The model under review builds one solid part; all positions refer to its coordinate system, in mm. Face numbers are marked on the shaded views. A direction names the side the tool comes from. Give positions to 0.01 mm unless a question says otherwise; leave off trailing zeros. Order: outer loops, then holes, each group sorted by start corner. A loop starts at its lowest first (then second) coordinate and runs counter-clockwise, first axis right, second up. Notation, with made-up numbers: (52.25, 61.5) -> (70.25, 61.5) arc R21 cw to (70.25, 74.5) -> close; hole circle Ø7 at (39, 41.5). An arc over 180 degrees is marked (long way). Use one line per item in the form item = value.
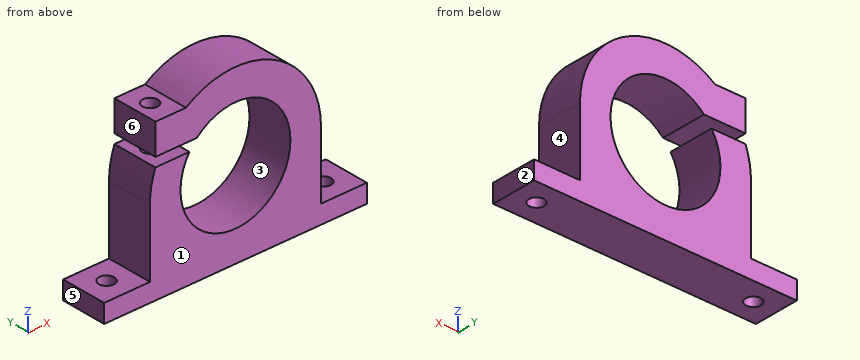
```python
from build123d import *

# Parameters (mm, degrees)
F1_DEPTH = 7.5
F2_R     = 2.5
F3_DEPTH = 6
F4_R     = 2.5
F5_DEPTH = 18


with BuildPart() as f1:
    # F0 (on Front) → F1 (new body, symmetric)
    with BuildSketch(Plane.XZ):
        with BuildLine():
            ThreePointArc((28, 0), (12.841967, 24.881396), (-16.220278, 22.823291))
            Line((-16.220278, 22.823291), (-26.220278, 22.823291))
            Line((-26.220278, 22.823291), (-26.220278, 12.823291))
            Line((-26.220278, 12.823291), (-12.631834, 12.823291))
            ThreePointArc((-12.631834, 12.823291), (13.938464, -11.389434), (-15.083201, 9.823291))
            Line((-15.083201, 9.823291), (-26.220278, 9.823291))
            ThreePointArc((-26.220278, 9.823291), (-27.551477, 4.991604), (-28, 0))
            Line((-28, 0), (-28, -22))
            Line((-28, -22), (-43, -22))
            Line((-43, -22), (-43, -28))
            Line((-43, -28), (43, -28))
            Line((43, -28), (43, -22))
            Line((43, -22), (28, -22))
            Line((28, -22), (28, 0))
        make_face()
    extrude(amount=F1_DEPTH, both=True)

    # F2 (on face) → F3 (cut, through all)
    with BuildSketch(Plane.XY.offset(-22)):
        with Locations((-35.5, 0)):
            Circle(F2_R)
        with Locations((35.5, 0)):
            Circle(F2_R)
    extrude(amount=-F3_DEPTH, mode=Mode.SUBTRACT)

    # F4 (on face) → F5 (cut)
    with BuildSketch(Plane.XY.offset(22.823291)):
        with Locations((-21.220278, 0)):
            Circle(F4_R)
    extrude(amount=-F5_DEPTH, mode=Mode.SUBTRACT)


solid = f1.part
```
1. For L1, parallel to Y at x = 35.5, z = -23.95; L2, parallel to Z at x = -16, y = -4; L3, parallel to Z at x = 4, y = 3.5, list the stretches that pass through material, from the lowest coordinate up.
Values:
L1 = -7.5 to -2.5, 2.5 to 7.5
L2 = -28 to -8.25, 8.25 to 9.82, 12.82 to 22.98
L3 = -28 to -17.55, 17.55 to 27.71
2. Add section D-D on z = 7. Give the boundary of the cut face in (x, y).
Values:
outline = (-27.11, -7.5) -> (-16.58, -7.5) -> (-16.58, 7.5) -> (-27.11, 7.5) -> close; (16.58, -7.5) -> (27.11, -7.5) -> (27.11, 7.5) -> (16.58, 7.5) -> close; hole circle Ø5 at (-21.22, 0)
3. Add section A-A on y = 0. Count the separate pieces of the cut face and the enclosed holes in it, then the cut area to 3 significant figures.
Values:
separate_pieces = 4
enclosed_holes = 0
area = 1,840 mm^2
4. Add section C-C on x = 35.5. Give the boundary of the cut face in (y, z), then the cut area to 3 significant figures.
Values:
outline = (-7.5, -28) -> (-2.5, -28) -> (-2.5, -22) -> (-7.5, -22) -> close; (2.5, -28) -> (7.5, -28) -> (7.5, -22) -> (2.5, -22) -> close
area = 60.0 mm^2
5. Add section B-B on z = -17. Give the boundary of the cut face in (x, y), then the cut area to 3 significant figures.
Values:
outline = (-28, -7.5) -> (-5.92, -7.5) -> (-5.92, 7.5) -> (-28, 7.5) -> close; (5.92, -7.5) -> (28, -7.5) -> (28, 7.5) -> (5.92, 7.5) -> close
area = 663 mm^2
6. For pin 1 Ø4.5 at (y, z) = (-3.5, -12.5) entering from +X; pin 2 Ø8 at (y, z) = (-3, 20) entering from -X; pin 3 Ø4.5 at (x, y) = (39, -2) entering from +Z; pin 4 Ø6 at (x, y) = (-2.5, -2.5) entering from +Z, all flat-tipped, find the tip position at first contact; note any pin that passes through.
Values:
pin_1 = 28
pin_2 = -26.22
pin_3 = -22
pin_4 = 28
7. Tool access review of the marked faces 4, 5 and 6: name each direction out of +Z, -Z, +X, -X, +Y, -Y from which nothing blocks a thin tool from reaching the whole face with its end or side.
Values:
face_4 = +Z, +X, +Y, -Y
face_5 = +Z, -Z, -X, +Y, -Y
face_6 = +Z, -X, +Y, -Y
8. The part is to be moulded in two halves that separate along X. For the marked faces 1, 2 and 3, say which applies: +X half, -X half, draft (parallel to the pull), parting line (faces both ways), or undercut.
Values:
face_1 = draft
face_2 = +X half
face_3 = undercut
